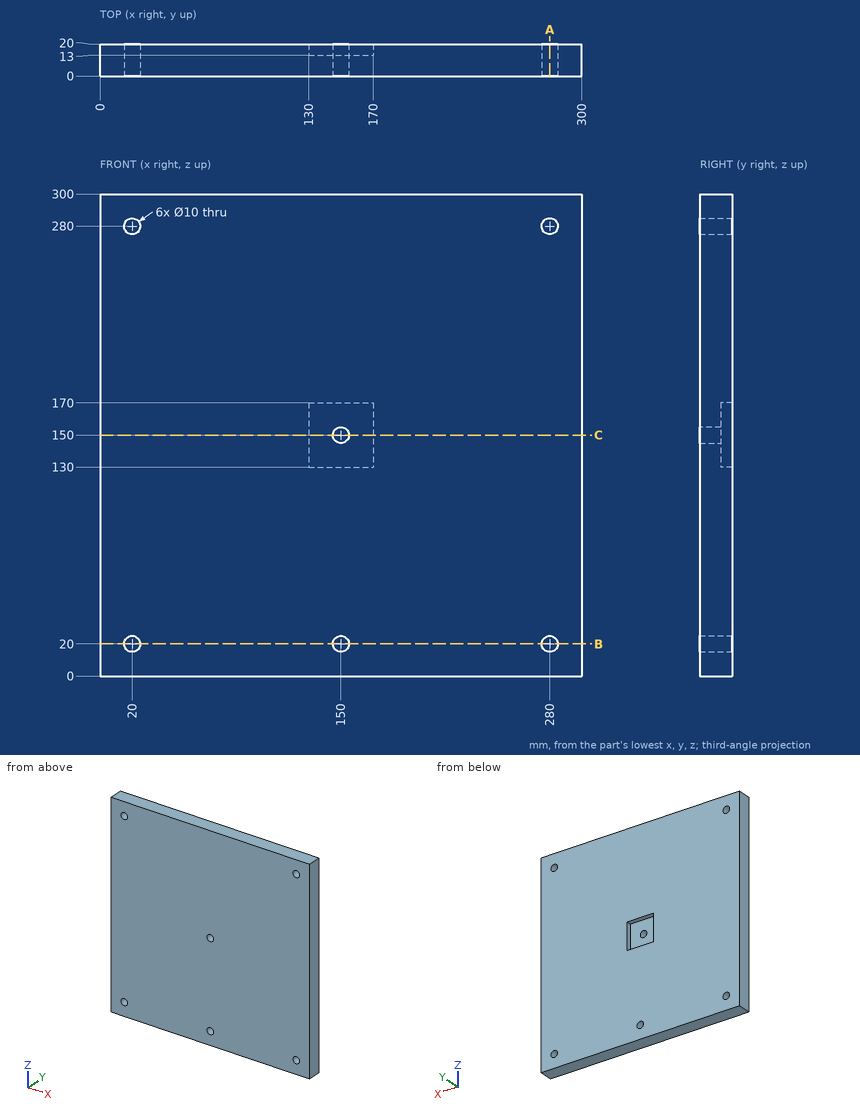
Geometry check sheet. Reference: drawing and pictorial views, mm from the part's lowest x, y, z. Give positions to 0.01 mm unless a question says otherwise; leave off trailing zeros. Order: outer loops, then holes, each group sorted by start corner. A loop starts at its lowest first (then second) coordinate and runs counter-clockwise, first axis right, second up. Notation, with made-up numbers: M -26.75,75 L -3.75,75 A15 ccw -3.75,93 Z; hole C 54,39 d4. An arc over 180 degrees is marked long. Answer in a Markdown table with one row per item. Add a question column.
Q1. Thickness scan on L1, parallel to Z at x = 150, y = 7; L2, parallel to X at y = 11.75, z = 280; L3, parallel to X at y = 5, z = 20. Record the ranges inside material, lowest first.
Q2. Sectioned sample at A-A, the plane x = 280. Record the boundary of the cut face in (y, z).
Q3. Sectioned sample at C-C, the plane z = 150. Record the boundary of the cut face in (x, y).
Q4. Sectioned sample at B-B, the plane z = 20. Record the boundary of the cut face in (x, y), and give its area (3 significant figures).
Q5. Gauge pin test, flat end, axial feed: pin 1 Ø12 at (x, z) = (157, 151) entering from +Y. Record the tip position at first contact, or that the pin passes through.
Verdict:
| question | item | result |
|---|---|---|
| 1 | L1 | 0 to 15, 25 to 145, 155 to 300 |
| 1 | L2 | 0 to 15, 25 to 275, 285 to 300 |
| 1 | L3 | 0 to 15, 25 to 145, 155 to 275, 285 to 300 |
| 2 | outline | M 0,0 L 20,0 L 20,15 L 0,15 Z; M 0,25 L 20,25 L 20,275 L 0,275 Z; M 0,285 L 20,285 L 20,300 L 0,300 Z |
| 3 | outline | M 0,0 L 145,0 L 145,13 L 130,13 L 130,20 L 0,20 Z; M 155,0 L 300,0 L 300,20 L 170,20 L 170,13 L 155,13 Z |
| 4 | outline | M 0,0 L 15,0 L 15,20 L 0,20 Z; M 25,0 L 145,0 L 145,20 L 25,20 Z; M 155,0 L 275,0 L 275,20 L 155,20 Z; M 285,0 L 300,0 L 300,20 L 285,20 Z |
| 4 | area | 5,400 mm² |
| 5 | pin 1 | y = 13 |
